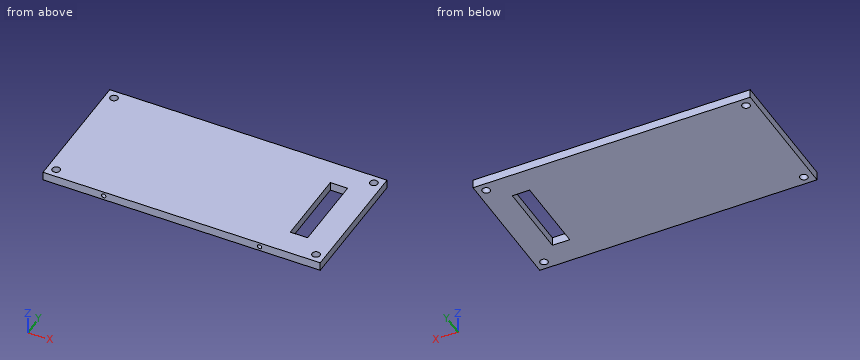
from build123d import *

# Parameters (mm, degrees)
SKETCH_W       = 160
SKETCH_H       = 75
PAD_DEPTH      = 5
SKETCH001_R    = 2.25
HOLE_DEPTH     = 5.001
SKETCH002_R    = 1.25
HOLE001_DEPTH  = 25
HOLE001_TIPS_R = 1.25
SKETCH003_W    = 10
SKETCH003_H    = 45
POCKET_DEPTH   = 5


with BuildPart() as part:
    # Sketch → Pad (new body)
    with BuildSketch(Plane.XY):
        Rectangle(SKETCH_W, SKETCH_H)
    extrude(amount=PAD_DEPTH)

    # Sketch001 (on Face5 of Pad) → Hole (cut, through all)
    with BuildSketch(Plane(origin=(0, 0, 0), x_dir=(1, 0, 0), z_dir=(0, 0, -1))):
        with Locations((-75, 32.5)):
            Circle(SKETCH001_R)
        with Locations((75, 32.5)):
            Circle(SKETCH001_R)
        with Locations((75, -32.5)):
            Circle(SKETCH001_R)
        with Locations((-75, -32.5)):
            Circle(SKETCH001_R)
    extrude(amount=-HOLE_DEPTH, mode=Mode.SUBTRACT)

    # Sketch002 (on Face6 of Hole) → Hole001 (cut)
    with BuildSketch(Plane.XZ.offset(37.5)):
        with Locations((-45, 2.5)):
            Circle(SKETCH002_R)
        with Locations((45, 2.5)):
            Circle(SKETCH002_R)
    extrude(amount=-HOLE001_DEPTH, mode=Mode.SUBTRACT)

    # Hole001 tips → Hole001 tip 1 section 0
    with BuildSketch(Plane.XZ.offset(12.5), mode=Mode.PRIVATE) as hole001_tip_1_s0:
        with Locations((-45, 2.5)):
            Circle(HOLE001_TIPS_R)
    loft([hole001_tip_1_s0.sketch, Vertex(-45, -11.748924, 2.5)], mode=Mode.SUBTRACT)

    # Hole001 tips → Hole001 tip 2 section 0
    with BuildSketch(Plane.XZ.offset(12.5), mode=Mode.PRIVATE) as hole001_tip_2_s0:
        with Locations((45, 2.5)):
            Circle(HOLE001_TIPS_R)
    loft([hole001_tip_2_s0.sketch, Vertex(45, -11.748924, 2.5)], mode=Mode.SUBTRACT)

    # Sketch003 (on Face4 of Hole001) → Pocket (cut)
    with BuildSketch(Plane(origin=(0, 0, 0), x_dir=(1, 0, 0), z_dir=(0, 0, -1))):
        with Locations((60, 0)):
            Rectangle(SKETCH003_W, SKETCH003_H)
    extrude(amount=-POCKET_DEPTH, mode=Mode.SUBTRACT)


solid = part.part
Model file for the job. Use its own axes, mm. Round coordinates to 2 decimals unless told otherwise and drop trailing zeros. Order: outer loops, then holes, each group sorted by start corner. A loop starts at its lowest first (then second) coordinate and runs counter-clockwise, first axis right, second up.
(1) Band-saw the part on D-D (y = -15). List the corners of the cut face in (x, z), then the cut area to 3 significant figures.
(2) Band-saw the part on C-C (x = -75). List the corners of the cut face in (y, z), then the cut area to 3 significant figures.
(3) Band-saw the part on A-A (y = 15). List the corners of the cut face in (x, z), then the cut area to 3 significant figures.
(4) Band-saw the part on B-B (y = -32.5). List the corners of the cut face in (x, z), then the cut area to 3 significant figures.
(5) Drill centre lines: line 1 (Y direction, x = 75, z = 2.45); line 2 (X direction, y = 32.5, z = 3.2); line 3 (Z direction, x = 45, y = -28). Where is each one in solid material? Low to high.
Verdict:
1. outline: (-80, 0) - (55, 0) - (55, 5) - (-80, 5) - close; (65, 0) - (80, 0) - (80, 5) - (65, 5) - close; hole circle Ø2.5 at (-45, 2.5); hole circle Ø2.5 at (45, 2.5)
1. area: 740 mm2
2. outline: (-37.5, 0) - (-34.75, 0) - (-34.75, 5) - (-37.5, 5) - close; (-30.25, 0) - (30.25, 0) - (30.25, 5) - (-30.25, 5) - close; (34.75, 0) - (37.5, 0) - (37.5, 5) - (34.75, 5) - close
2. area: 330 mm2
3. outline: (-80, 0) - (55, 0) - (55, 5) - (-80, 5) - close; (65, 0) - (80, 0) - (80, 5) - (65, 5) - close
3. area: 750 mm2
4. outline: (-80, 0) - (-77.25, 0) - (-77.25, 5) - (-80, 5) - close; (-72.75, 0) - (72.75, 0) - (72.75, 5) - (-72.75, 5) - close; (77.25, 0) - (80, 0) - (80, 5) - (77.25, 5) - close; hole circle Ø2.5 at (-45, 2.5); hole circle Ø2.5 at (45, 2.5)
4. area: 745 mm2
5. line 1: y = -37.5 to -34.75, -30.25 to 30.25, 34.75 to 37.5
5. line 2: x = -80 to -77.25, -72.75 to 72.75, 77.25 to 80
5. line 3: z = 0 to 1.25, 3.75 to 5
